Build history of the part. All positions in model axes, mm. Face numbers are marked on the shaded views. A direction names the side the tool comes from. Give positions to 0.01 mm unless a question says otherwise; leave off trailing zeros. Write each loop counter-clockwise with the first axis right and the second up, starting at its lowest first coordinate (ties: lowest second). Pieces come first, ordered by that corner, then holes. Notation, with made-up numbers: (11, -37.75) -> (57, -37.75) arc R13 ccw to (57, -30.75) -> close; hole circle Ø11 at (79, 36). An arc over 180 degrees is marked (long way). Put each result on its own line as item: value. Start each with the question number.
Item 1: Two-plate mould, pull along Y, no slides. Class the marked faces 1, 2 and 3: pulls with the +Y half, pulls with the -Y half, needs draft (parallel to the pull), parting line crosses it, or undercut.
Item 2: Drill centre lines: line 1 along Z through (x, y) = (-44.5, -9); line 2 along X through (y, z) = (1, 10); line 3 along Y through (x, z) = (0.5, 6.5). Where is each one in solid material? Low to high.
Item 3: Flat gauge pins, fed straight in: pin 1 Ø5 at (x, y) = (-21, -19.5) entering from +Z; pin 2 Ø1.5 at (y, z) = (49.5, 81.5) entering from +X; pin 3 Ø4 at (x, z) = (-49.5, 75.5) entering from +Y. Where does each tip first touch, or does it go through?
Item 4: Tool access for the marked faces 4, 5 and 6: list every direction of +Z, -Z, +X, -X, +Y, -Y with a clear straight run to the whole face (end or side of a thin tool).
Item 5: Slice it at C-C, the plane y = 22.5. List the corners of the cut face in (x, z), plus the area to 3 significant figures.
Item 6: Slice it at D-D, the plane z = 42. List the corners of the cut face in (x, y).
Item 7: Slice it at B-B, the plane y = 37.5. List the corners of the cut face in (x, z).
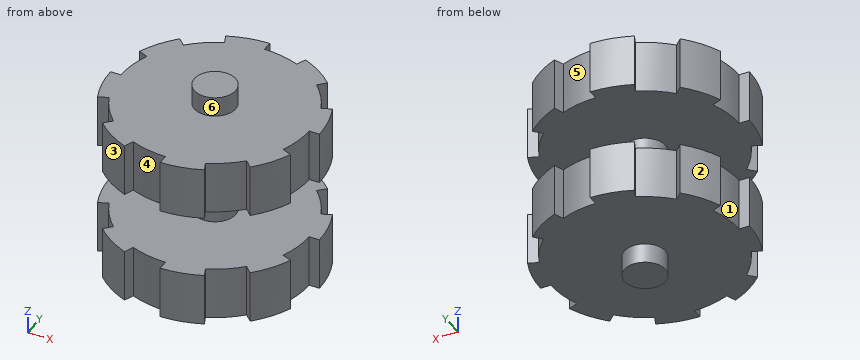
Autodesk Inventor part; units mm, degrees
ref_plane "YZ Plane" through (0, 0, 0) normal (1, 0, 0) x (0, 1, 0)
ref_plane "XZ Plane" through (0, 0, 0) normal (0, 1, 0) x (-1, 0, 0)
ref_plane "XY Plane" through (0, 0, 0) normal (0, 0, 1) x (1, 0, 0)
sketch "Esboço1" plane through (0, 0, 0) normal (1, 0, 0) x (0, 1, 0)
  line L0 (0, 0) -> (0, 100)
  line L1 (0, 100) -> (10, 100)
  line L2 (10, 100) -> (10, 90.4)
  line L3 (10, 90.4) -> (50.8, 90.4)
  line L4 (50.8, 90.4) -> (50.8, 65)
  line L5 (50.8, 65) -> (10, 65)
  line L6 (10, 65) -> (10, 35)
  line L7 (10, 35) -> (50.8, 35)
  line L8 (50.8, 35) -> (50.8, 9.6)
  line L9 (50.8, 9.6) -> (10, 9.6)
  line L10 (10, 9.6) -> (10, 0)
  line L11 (10, 0) -> (0, 0)
  line L12 (0, 50) -> (10, 50)
  dimension "d0" = 10
  dimension "d1" = 100
  dimension "d2" = 25.4
  dimension "d3" = 25.4
  dimension "d4" = 15
  dimension "d5" = 15
  dimension "d6" = 50.8
revolve "Revolução1" add sketch "Esboço1" angle 360 about axis through (0, 0, 0) along (0, 0, 1)
thread "Rosca1"
thread "Rosca2"
sketch "Esboço4" plane through (0, 0, 90.4) normal (0, 0, 1) x (1, 0, 0)
  circle A0 centre (0, 0) radius 10
  circle A1 centre (0, 0) radius 50.8
  line L0 (0, 0) -> (0, 50.8)
  line L1 (0, 0) -> (0, -50.8)
  line L2 (0, 0) -> (50.8, 0)
  line L3 (0, 0) -> (-50.8, 0)
  line L4 (0, 0) -> (-35.921, 35.921)
  line L5 (0, 0) -> (-19.4403, 46.9331)
  line L6 (0, 0) -> (-46.9331, 19.4403)
  line L7 (0, 0) -> (35.921, 35.921)
  line L8 (0, 0) -> (19.4403, 46.9331)
  line L9 (0, 0) -> (46.9331, 19.4403)
  line L10 (0, 0) -> (-35.921, -35.921)
  line L11 (0, 0) -> (-19.4403, -46.9331)
  line L12 (0, 0) -> (-46.9331, -19.4403)
  line L13 (0, 0) -> (19.4403, -46.9331)
  line L14 (0, 0) -> (35.921, -35.921)
  line L15 (0, 0) -> (46.9331, -19.4403)
  circle A2 centre (0, 0) radius 45.8
  point P0 (-5, 45.5263)
  point P1 (-45.8, 0)
  point P2 (0, -45.8)
  point P3 (45.8, 0)
  point P4 (0, 45.8)
  point P5 (-42.3137, -17.5269)
  point P6 (17.5269, -42.3137)
  point P7 (42.3137, 17.5269)
  point P8 (-17.5269, 42.3137)
  point P9 (17.5269, 42.3137)
  point P10 (42.3137, -17.5269)
  point P11 (32.3855, 32.3855)
  point P12 (32.3855, -32.3855)
  point P13 (-32.3855, 32.3855)
  point P14 (-42.3137, 17.5269)
  point P15 (-32.3855, -32.3855)
  point P16 (-17.5269, -42.3137)
  dimension "d21" = 45
  dimension "d22" = 22.5
  dimension "d23" = 22.5
extrude "Extrusão3" cut sketch "Esboço4" against normal up to surface (80.8 mm away) contours L2 A1 L15 A2 | A2 L7 A1 L9 | L14 A1 L13 A2 | L0 A1 L8 A2 | L1 A1 L11 A2 | L3 A1 L6 A2 | L4 A1 L5 A2 | L10 A1 L12 A2
equation "\"d3\" = d2"
equation "\"d5\" = d4"
equation "\"d22\" = 0.5 * d21"
equation "\"d23\" = d22"
properties part number "Coletor - Hand"
Values follow:
1. face 1: undercut
1. face 2: pulls with the +Y half
1. face 3: pulls with the -Y half
2. line 1: 9.6 to 35, 65 to 90.4
2. line 2: -45.79 to 50.79
2. line 3: -9.99 to 9.99
3. pin 1: z = 90.4
3. pin 2: x = 0
3. pin 3: y = 0
4. face 4: +Z, -Z, -Y
4. face 5: +Z, -Z, +Y
4. face 6: +Z
5. outline: (-45.55, 9.6) -> (39.89, 9.6) -> (39.89, 35) -> (-45.55, 35) -> close; (-45.55, 65) -> (39.89, 65) -> (39.89, 90.4) -> (-45.55, 90.4) -> close
5. area: 4,340 mm2
6. outline: circle Ø20 at (0, 0)
7. outline: (-26.29, 9.6) -> (34.27, 9.6) -> (34.27, 35) -> (-26.29, 35) -> close; (-26.29, 65) -> (34.27, 65) -> (34.27, 90.4) -> (-26.29, 90.4) -> close
